Source: CAD feature listing. Evaluate the final solid. Frame: model axes, mm. A direction names the side the tool comes from. Round coordinates to 2 decimals unless told otherwise and drop trailing zeros. Write each loop counter-clockwise with the first axis right and the second up, starting at its lowest first coordinate (ties: lowest second). Pieces come first, ordered by that corner, then holes. Notation, with made-up numbers: M 85,31 L 141,31 A23 cw 141,60 Z; hole C 68,10 d2. An arc over 180 degrees is marked long. Answer in a Markdown table with one row per item. Add a question column.
Item 1: Contact query for flat-ended pins moving along their axis: pin 1 (3 mm diameter, centred on x = 2, y = 2, fed in from +Z); pin 2 (1 mm diameter, centred on x = 0, y = -1, fed in from -Z); pin 3 (1 mm diameter, centred on x = -1.5, z = 12.5, fed in from -Y); pin 4 (0.8 mm diameter, centred on y = 0.5, z = 1, fed in from -X). Output: stop coordinate, or through.
Item 2: Cut plane A-A on z = 14. Return loops of the section in (x, y).
Item 3: Mould query, pull axis X, two halves, no side actions, for faces 1 (the face through (-0.45, 0, 1)), 2 (the face through (0.37, 2.85, 2)), 3 (the face through (0, 0, 17.7)). Classes: released by +X, released by -X, zero draft, split by the parting line, or undercut.
Item 4: Set-up query: faces 4 (the face through (0, 0, 1.5)), 5 (the face through (-1.2, -1.2, 2.2)). Return all of +Z, -Z, +X, -X, +Y, -Y with unobstructed straight access to the full face (end or side cutting, diameter ignored); none if empty.
Item 5: Material intervals for probe 1 along Z at (x, y) = (-0.2, -1.9); probe 2 along Y at (x, z) = (-1.05, 8); probe 3 along X at (y, z) = (-1.2, 2.5), sorted ascending.
from build123d import *

# Parameters (mm, degrees)
ESBO_O1_R                = 1.5
RESSALTO_EXTRUS_O1_DEPTH = 17.7
ESBO_O2_R                = 2.875
RESSALTO_EXTRUS_O2_DEPTH = 2.2
FILETE1_R                = 1.8
ESBO_O3_W                = 0.9
ESBO_O3_H                = 6.121542056
CORTE_EXTRUS_O1_DEPTH    = 1.5
CHANFRO1_SIZE            = 0.2


with BuildPart() as part:
    # Esboço1 → Ressalto-extrusão1 (new body)
    with BuildSketch(Plane.XY):
        Circle(ESBO_O1_R)
    extrude(amount=RESSALTO_EXTRUS_O1_DEPTH)

    # Esboço2 → Ressalto-extrusão2 (add)
    with BuildSketch(Plane(origin=(0, 0, 0), x_dir=(-1, 0, 0), z_dir=(0, 0, -1))):
        Circle(ESBO_O2_R)
    extrude(amount=-RESSALTO_EXTRUS_O2_DEPTH)

    # Filete1
    filete1_edges = [part.edges().sort_by_distance(p)[0] for p in [
        (2.875, 0, 0),
    ]]
    fillet(filete1_edges, radius=FILETE1_R)

    # Esboço3 → Corte-extrusão1 (cut)
    with BuildSketch(Plane(origin=(0, 0, 0), x_dir=(-1, 0, 0), z_dir=(0, 0, -1))):
        Rectangle(ESBO_O3_W, ESBO_O3_H)
    extrude(amount=-CORTE_EXTRUS_O1_DEPTH, mode=Mode.SUBTRACT)

    # Chanfro1
    chanfro1_edges = [part.edges().sort_by_distance(p)[0] for p in [
        (-1.5, 0, 17.7),
    ]]
    chamfer(chanfro1_edges, length=CHANFRO1_SIZE)


solid = part.part
Results below:
| question | item | result |
|---|---|---|
| 1 | pin 1 | z = 17.67 |
| 1 | pin 2 | z = 0 |
| 1 | pin 3 | y = -1.12 |
| 1 | pin 4 | x = -2.8 |
| 2 | outline | C 0,0 d3 |
| 3 | face 1 | undercut |
| 3 | face 2 | split by the parting line |
| 3 | face 3 | zero draft |
| 4 | face 4 | -Z, +Y, -Y |
| 4 | face 5 | +Z |
| 5 | probe 1 | 1.5 to 2.2 |
| 5 | probe 2 | -1.07 to 1.07 |
| 5 | probe 3 | -0.9 to 0.9 |
